Geometry: final body of the model. Coordinates: model frame, mm. Give positions to 0.01 mm unless a question says otherwise; leave off trailing zeros. Use a Markdown table: item, result. Add a question column.
1) Pin query (flat end, axial travel): pin 1 (2.5 mm diameter, centred on x = 6.5, y = 3, fed in from +Z); pin 2 (1.4 mm diameter, centred on x = 502, y = 2.5, fed in from -Z); pin 3 (2.5 mm diameter, centred on x = 499, y = 3, fed in from +Z). Return the tip coordinate at first contact, or that it passes through.
2) Line query: line 1 (Z direction, x = 10.16, y = 3.15); line 2 (X direction, y = 3.65, z = 50.8) (1 decimal); line 3 (Z direction, x = 38.1, y = 2.9) (3 decimals). Output: solid intervals per line, ascending.
3) Draft query along X for faces 1 (the cylindrical face through (19.048, 2.348, 31.945)), 2 (the cylindrical face through (500.693, 2.348, 50.591)), 3 (the flat face through (250, 4.762, 31)), 4 (the cylindrical face through (500.693, 2.348, 12.491)). Return one class per face: +X half, -X half, draft (parallel to the pull), parting line (faces both ways), or undercut.
4) Section A-A on y = 3.4. State how many separate pieces and enclosed holes the cut face has, then the cut area to 3 significant figures.
```python
from build123d import *

# Parameters (mm, degrees)
SKETCH1_R           = 4.7625
SKETCH1_R_2         = 1.905
BOSS_EXTRUDE1_DEPTH = 4.7625


with BuildPart() as part:
    # Sketch1 → Boss-Extrude1 (new body)
    with BuildSketch(Plane(origin=(0, 0, 0), x_dir=(1, 0, 0), z_dir=(0, 1, 0))):
        with BuildLine():
            Line((10.16, 0), (253.0475, 0))
            Line((253.0475, 0), (253.0475, -63.5))
            Line((253.0475, -63.5), (10.16, -63.5))
            ThreePointArc((10.16, -63.5), (2.975795103, -60.524204897), (0, -53.34))
            Line((0, -53.34), (0, -40.64))
            Line((0, -40.64), (10.16, -40.64))
            ThreePointArc((10.16, -40.64), (19.05, -31.75), (10.16, -22.86))
            Line((10.16, -22.86), (0, -22.86))
            Line((0, -22.86), (0, -10.16))
            ThreePointArc((0, -10.16), (2.975795103, -2.975795103), (10.16, 0))
        make_face()
        with Locations((10.16, -50.8)):
            Circle(SKETCH1_R, mode=Mode.SUBTRACT)
        with Locations((10.16, -12.7)):
            Circle(SKETCH1_R, mode=Mode.SUBTRACT)
        with Locations((38.1, -50.8)):
            Circle(SKETCH1_R_2, mode=Mode.SUBTRACT)
        with Locations((38.1, -12.7)):
            Circle(SKETCH1_R_2, mode=Mode.SUBTRACT)
    boss_extrude1 = extrude(amount=BOSS_EXTRUDE1_DEPTH)

    # Mirror1: Boss-Extrude1 across plane
    add(boss_extrude1.mirror(Plane(origin=(253.0475, 4.7625, 63.5), x_dir=(0, 0, 1), z_dir=(-1, 0, 0))))


solid = part.part
```
Found:
| question | item | result |
|---|---|---|
| 1 | pin 1 | z = 63.21 |
| 1 | pin 2 | z = 1.53 |
| 1 | pin 3 | z = 63.34 |
| 2 | line 1 | 0 to 7.94, 17.46 to 22.86, 40.64 to 46.04, 55.56 to 63.5 |
| 2 | line 2 | 0 to 5.4, 14.9 to 36.2, 40 to 466.1, 469.9 to 491.2, 500.7 to 506.1 |
| 2 | line 3 | 0 to 10.795, 14.605 to 48.895, 52.705 to 63.5 |
| 3 | face 1 | -X half |
| 3 | face 2 | undercut |
| 3 | face 3 | draft |
| 3 | face 4 | undercut |
| 4 | separate pieces | 1 |
| 4 | enclosed holes | 8 |
| 4 | area | 31,100 mm² |
